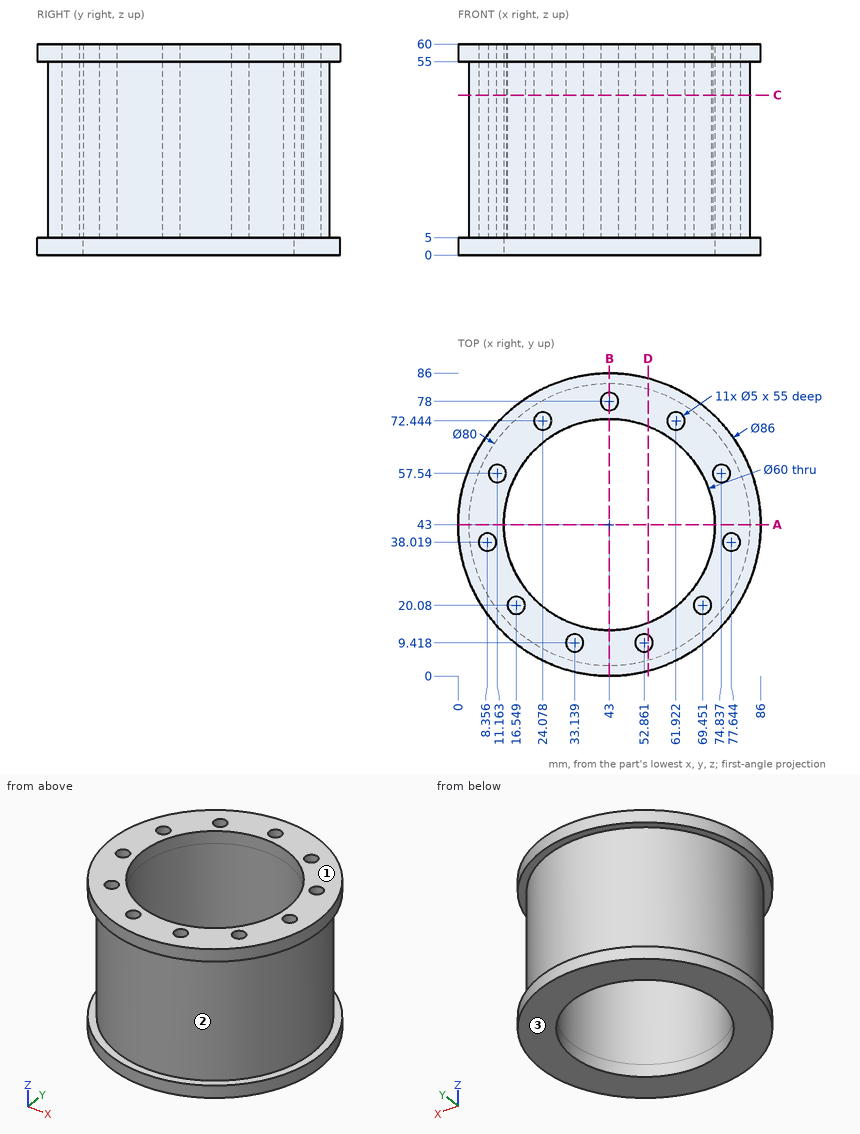
Geometry check sheet. Reference: drawing and pictorial views, mm from the part's lowest x, y, z. Round coordinates to 2 decimals unless told otherwise and drop trailing zeros. Order: outer loops, then holes, each group sorted by start corner. A loop starts at its lowest first (then second) coordinate and runs counter-clockwise, first axis right, second up. Notation, with made-up numbers: (-16.5, -38.5) -> (-1.5, -38.5) arc R22 cw to (-1.5, -15.5) -> close; hole circle Ø5 at (62.5, -18). An arc over 180 degrees is marked (long way). One line per item, written item: value. Start each with the question number.
Q1. Mould release check, pull along Z, two halves, no side actions. Record for the marked faces 1, 2 and 3: pulls with the +Z half, pulls with the -Z half, needs draft (parallel to the pull), parting line crosses it, or undercut.
Q2. Cross-section at C-C (z = 45.5). Give the number of separate pieces and of enclosed holes in the cut face, and give its area (3 significant figures).
Q3. Thickness scan on line 1 (Y direction, x = 43, z = 58.6); line 2 (Y direction, x = 43, z = 37); line 3 (X direction, y = 57.5, z = 47) (1 decimal). Record the ranges inside material, lowest first.
Q4. Cross-section at B-B (x = 43). Record the boundary of the cut face in (y, z).
Q5. Gauge pin test, flat ends, axial feed: pin 1 Ø1 at (x, z) = (22, 10.5) entering from +Y; pin 2 Ø4 at (x, z) = (70.5, 43.5) entering from -Y; pin 3 Ø2.5 at (x, y) = (70.5, 20.5) entering from +Z. Record the tip position at first contact, or that the pin passes through.
Q6. Cross-section at D-D (x = 54). Record the boundary of the cut face in (y, z), and give its area (3 significant figures).
Q7. Cross-section at A-A (y = 43). Record the boundary of the cut face in (x, z), and give its area (3 significant figures).
Completed:
1. face 1: pulls with the +Z half
1. face 2: undercut
1. face 3: pulls with the -Z half
2. separate pieces: 1
2. enclosed holes: 12
2. area: 1,980 mm²
3. line 1: y = 0 to 13, 73 to 75.5, 80.5 to 86
3. line 2: y = 3 to 13, 73 to 75.5, 80.5 to 83
3. line 3: x = 5.7 to 8.7, 13.7 to 16.7, 69.3 to 72.3, 77.3 to 80.3
4. outline: (0, 0) -> (13, 0) -> (13, 60) -> (0, 60) -> (0, 55) -> (3, 55) -> (3, 5) -> (0, 5) -> close; (73, 0) -> (86, 0) -> (86, 5) -> (83, 5) -> (83, 55) -> (86, 55) -> (86, 60) -> (80.5, 60) -> (80.5, 5) -> (75.5, 5) -> (75.5, 60) -> (73, 60) -> close
5. pin 1: stops at y = 77.35
5. pin 2: stops at y = 12.18
5. pin 3: stops at z = 5
6. outline: (1.43, 0) -> (15.09, 0) -> (15.09, 60) -> (11.64, 60) -> (11.64, 5) -> (7.19, 5) -> (7.19, 60) -> (1.43, 60) -> (1.43, 55) -> (4.54, 55) -> (4.54, 5) -> (1.43, 5) -> close; (70.91, 0) -> (84.57, 0) -> (84.57, 5) -> (81.46, 5) -> (81.46, 55) -> (84.57, 55) -> (84.57, 60) -> (70.91, 60) -> close
6. area: 1,080 mm²
7. outline: (0, 0) -> (13, 0) -> (13, 60) -> (0, 60) -> (0, 55) -> (3, 55) -> (3, 5) -> (0, 5) -> close; (73, 0) -> (86, 0) -> (86, 5) -> (83, 5) -> (83, 55) -> (86, 55) -> (86, 60) -> (73, 60) -> close
7. area: 1,260 mm²
